Autodesk Inventor part; units mm, degrees
ref_plane "Arbeitsebene1" through (0, 0, 0) normal (1, 0, 0) x (0, 1, 0)
ref_plane "XZ Plane" through (0, 0, 0) normal (0, 1, 0) x (-1, 0, 0)
ref_plane "XY Plane" through (0, 0, 0) normal (0, 0, 1) x (1, 0, 0)
sketch "Skizze1" plane through (0, 0, 0) normal (0, 0, 1) x (1, 0, 0)
  line L0 (-14, -11) -> (14, -11)
  line L1 (14, -11) -> (14, 11)
  line L2 (14, 11) -> (-14, 11)
  line L3 (-14, 11) -> (-14, -11)
  line L4 (-14, -11) -> (14, 11) construction
  line L5 (14, -11) -> (-14, 11) construction
  point P0 (0, 0)
  dimension "d0" = 28
  dimension "d1" = 22
extrude "Extrusion1" add sketch "Skizze1" along normal blind 6
sketch "Skizze2" plane through (-14, 11, 0) normal (0, 1, 0) x (1, 0, 0)
  circle A0 centre (14, -3) radius 5
  line L0 (0, 0) -> (0, -6)
  line L1 (28, 0) -> (0, 0)
  point P0 (14, 0)
  point P1 (0, -3)
  point P2 (14, 0)
  dimension "d4" = 10
extrude "Extrusion2" add sketch "Skizze2" along normal blind 80
ref_plane "Arbeitsebene1" through (0, 0, 0) normal (1, 0, 0) x (0, 1, 0)
sketch "Skizze3" plane through (0, 0, 0) normal (1, 0, 0) x (0, 1, 0)
  line L0 (91, -2) -> (91, 8)
  circle A0 centre (91, 3) radius 5
  point P0 (0, 0)
  dimension "d8" = 10
extrude "Extrusion3" add sketch "Skizze3" along normal mid plane 100
fillet "Rundung1" radius 2 2 edges at (50, 86, 3) (-50, 86, 3)
properties part number "Flutschlüssel"
The model under review builds one solid part; all positions refer to its coordinate system, in mm. A direction names the side the tool comes from. Coordinates: 2 decimals unless noted, no trailing zeros. Write each loop counter-clockwise with the first axis right and the second up, starting at its lowest first coordinate (ties: lowest second). Pieces come first, ordered by that corner, then holes. Notation, with made-up numbers: (-16.75, -7.5) - (16.25, -7.5) arc R17 ccw to (16.25, 12.5) - close; hole circle Ø7 at (75.5, 53.5). An arc over 180 degrees is marked (long way). Answer in a Markdown table with one row per item. Add a question column.
Q1. To check wall thickness, follow line 1 along X through (y, z) = (23, 3.25); line 2 along Y through (x, z) = (-40.5, 7); line 3 along X through (y, z) = (11.5, 0). State the ranges of each line that lie inside material, in increasing order. Write a range as from..to.
Q2. Consider section D-D on x = -28.5. Give the boundary of the cut face in (y, z).
Q3. Clearance check with flat-ended pins moving along their axes: pin 1 (5 mm diameter, centred on x = -7, z = 2, fed in from +Y); pin 2 (3 mm diameter, centred on y = 52, z = 3.5, fed in from +X); pin 3 (5 mm diameter, centred on x = 32, z = -0.5, fed in from -Y); pin 4 (2 mm diameter, centred on x = 2, z = -1.5, fed in from -Y). State where each tip first meets the part, or that it passes through.
Q4. Consider section A-A on x = -9.5. Give the boundary of the cut face in (y, z).
Q5. Consider section B-B on z = 3. Give the boundary of the cut face in (x, y).
Q6. Consider section C-C on y = 17. Give the boundary of the cut face in (x, z), then the cut area to 3 significant figures.
Q7. For faces 4 (the face through (0.67, 95.77, 4.5)), 5 (the face through (-14, 0, 3)), 6 (the face through (0, 0, 6)), 7 (the face through (14, 0, 3)), list the 3-axis set-ups (+Z, -Z, +X, -X, +Y, -Y) from which the entire face can be reached by the end or side of a thin tool; tool diameter is ignored.
Q8. Draft analysis for pull direction Y (two halves, no side actions). For faces 1 (the face through (0, -11, 3)), 2 (the face through (0, 0, 0)), 3 (the face through (-0.651, 50.44, 7.957)), state which applies: +Y half, -Y half, draft (parallel to the pull), parting line (faces both ways), or undercut.
Answers below:
| question | item | result |
|---|---|---|
| 1 | line 1 | -4.99..4.99 |
| 1 | line 2 | 88..94 |
| 1 | line 3 | -4..4 |
| 2 | outline | circle Ø10 at (91, 3) |
| 3 | pin 1 | y = 96 |
| 3 | pin 2 | x = 5 |
| 3 | pin 3 | y = 86.1 |
| 3 | pin 4 | y = 11 |
| 4 | outline | (-11, 0) - (11, 0) - (11, 6) - (-11, 6) - close; circle Ø10 at (91, 3) |
| 5 | outline | (-50, 88) arc R2 ccw to (-48, 86) - (-5, 86) - (-5, 11) - (-14, 11) - (-14, -11) - (14, -11) - (14, 11) - (5, 11) - (5, 86) - (48, 86) arc R2 ccw to (50, 88) - (50, 94) arc R2 ccw to (48, 96) - (-48, 96) arc R2 ccw to (-50, 94) - close |
| 6 | outline | circle Ø10 at (0, 3) |
| 6 | area | 78.5 mm² |
| 7 | face 4 | none |
| 7 | face 5 | +Z, -Z, -X, -Y |
| 7 | face 6 | +Z, +X, -X, -Y |
| 7 | face 7 | +Z, -Z, +X, -Y |
| 8 | face 1 | -Y half |
| 8 | face 2 | draft |
| 8 | face 3 | undercut |
